Job drawing, mm, ordinate dimensions from the low corner. One solid piece. Coordinates: 2 decimals unless noted, no trailing zeros. Write each loop counter-clockwise with the first axis right and the second up, starting at its lowest first coordinate (ties: lowest second). Pieces come first, ordered by that corner, then holes. Notation, with made-up numbers: (-20, -3) -> (5, -3) arc R15 cw to (5, 15) -> close; hole circle Ø10 at (-4.5, 37.25). An arc over 180 degrees is marked (long way). One line per question, with ' | ' between items. Start each with the question number.
Item 1: Probe probe 1 along X at (y, z) = (1.85, 3.5); probe 2 along Z at (x, y) = (86, 1.3); probe 3 along Z at (x, y) = (91, 1.15). List the from-to ranges inside material, lowest first. Write a range as [from, to].
Item 2: Saw through at B-B (x = 83). List the corners of the cut face in (y, z).
Item 3: Saw through at D-D (y = 1.65). Count the separate pieces of the cut face and the enclosed holes in it, and give its area (3 significant figures).
Item 4: Saw through at A-A (x = 22). List the corners of the cut face in (y, z), and give its area (3 significant figures).
Item 5: Saw through at C-C (z = 21). List the corners of the cut face in (x, y), and give its area (3 significant figures).
Item 6: Pin check, flat tips, straight feed: pin 1 (12 mm diameter, centred on x = 51.5, z = 55, fed in from -Y); pin 2 (1.5 mm diameter, centred on y = 1.5, z = 15, fed in from +X); pin 3 (0.9 mm diameter, centred on y = 1.5, z = 54, fed in from +X). Stop position of each tip, or through.
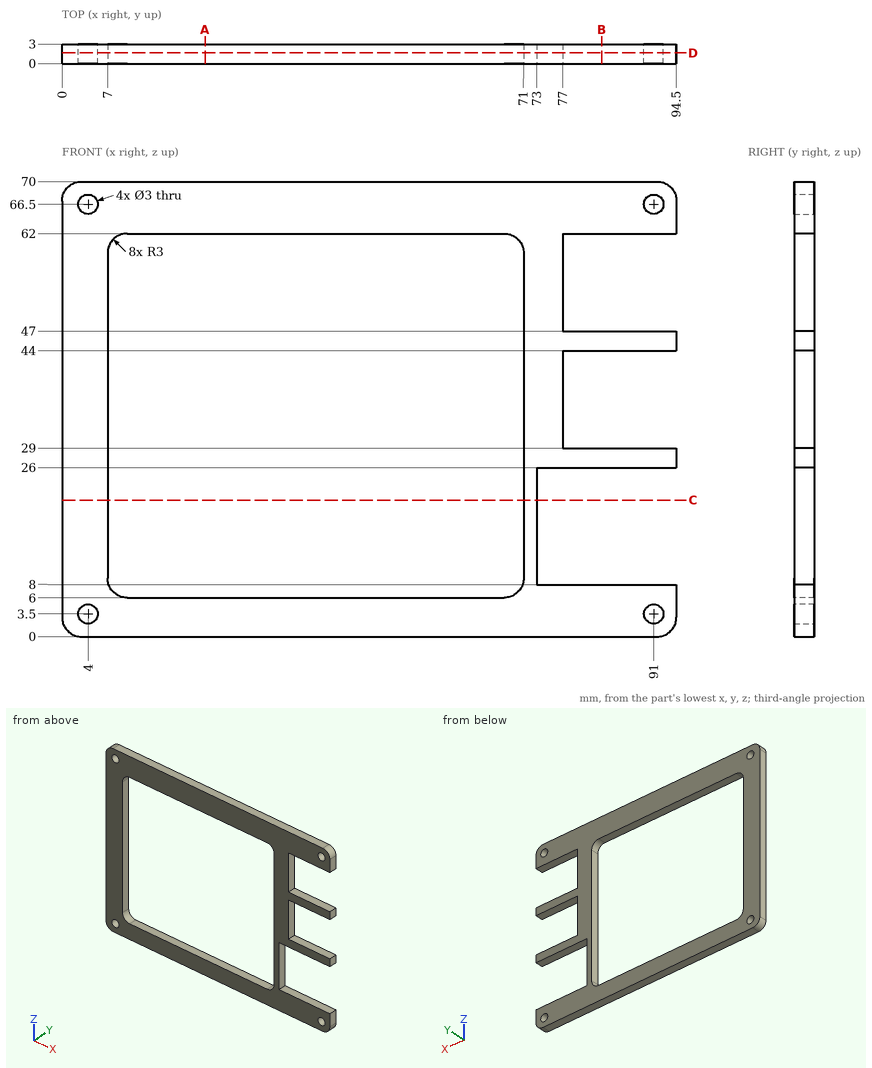
From the geometry:
1) probe 1: [0, 2.5], [5.5, 89.5], [92.5, 94.5] | probe 2: [0, 8], [26, 29], [44, 47], [62, 70] | probe 3: [0, 2], [5, 8], [26, 29], [44, 47], [62, 65], [68, 70]
2) outline: (0, 0) -> (3, 0) -> (3, 8) -> (0, 8) -> close; (0, 26) -> (3, 26) -> (3, 29) -> (0, 29) -> close; (0, 44) -> (3, 44) -> (3, 47) -> (0, 47) -> close; (0, 62) -> (3, 62) -> (3, 70) -> (0, 70) -> close
3) separate pieces: 1 | enclosed holes: 5 | area: 2,090 mm2
4) outline: (0, 0) -> (3, 0) -> (3, 6) -> (0, 6) -> close; (0, 62) -> (3, 62) -> (3, 70) -> (0, 70) -> close | area: 42.0 mm2
5) outline: (0, 0) -> (7, 0) -> (7, 3) -> (0, 3) -> close; (71, 0) -> (73, 0) -> (73, 3) -> (71, 3) -> close | area: 27.0 mm2
6) pin 1: through | pin 2: x = 73 | pin 3: x = 77
